from build123d import *

# Parameters (mm, degrees)
ESBO_O1_W                = 15
ESBO_O1_H                = 17
ESBO_O1_R                = 1
RESSALTO_EXTRUS_O1_DEPTH = 1.6
CHANFRO1_SIZE            = 2


with BuildPart() as part:
    # Esboço1 → Ressalto-extrusão1 (new body)
    with BuildSketch(Plane.XY):
        with Locations((2.895389518, -3.7)):
            Rectangle(ESBO_O1_W, ESBO_O1_H)
        with Locations((8.895389518, -3.7)):
            Circle(ESBO_O1_R, mode=Mode.SUBTRACT)
        with Locations((-3.104610482, -3.7)):
            Circle(ESBO_O1_R, mode=Mode.SUBTRACT)
    extrude(amount=RESSALTO_EXTRUS_O1_DEPTH)

    # Chanfro1
    chanfro1_edges = [part.edges().sort_by_distance(p)[0] for p in [
        (-4.604610482, 4.8, 0.8),
        (10.395389518, 4.8, 0.8),
        (10.395389518, -12.2, 0.8),
        (-4.604610482, -12.2, 0.8),
    ]]
    chamfer(chanfro1_edges, length=CHANFRO1_SIZE)


solid = part.part
Geometry check sheet. Reference: the model listing, model coordinates, mm. Round coordinates to 2 decimals unless told otherwise and drop trailing zeros. Order: outer loops, then holes, each group sorted by start corner. A loop starts at its lowest first (then second) coordinate and runs counter-clockwise, first axis right, second up. Notation, with made-up numbers: M 39.25,80.25 L 55.25,80.25 A5 ccw 55.25,88.25 Z; hole C 63.5,31 d6. An arc over 180 degrees is marked long. Answer in a Markdown table with one row per item. Add a question column.
Item 1: Material ranges on L1, parallel to X at y = -3.75, z = 0.4; L2, parallel to Y at x = -3.5, z = 0.1; L3, parallel to Y at x = -2.75, z = 0.35, recorded low to high. Write a range as [from, to].
Item 2: Sectioned sample at B-B, the plane x = 9.5. Enter the section's corners in (y, z).
Item 3: Sectioned sample at C-C, the plane y = -3.7. Enter the section's corners in (x, z).
Item 4: Draft check along Y on faces 1 (the face through (-2.15, -3.4, 0.79)), 2 (the face through (9.409, 3.786, 0.789)), 3 (the face through (3, -4, 0)). Enter one of: released by +Y, released by -Y, zero draft, split by the parting line, or undercut.
Item 5: Sectioned sample at A-A, the plane z = 0.7. Enter the section's corners in (x, y), plus the area to 3 significant figures.
Filled in:
| question | item | result |
|---|---|---|
| 1 | L1 | x = [-4.6, -4.1], [-2.11, 7.9], [9.89, 10.4] |
| 1 | L2 | y = [-11.3, -4.62], [-2.78, 3.9] |
| 1 | L3 | y = [-12.05, -4.64], [-2.76, 4.65] |
| 2 | outline | M -11.1,0 L -4.5,0 L -4.5,1.6 L -11.1,1.6 Z; M -2.9,0 L 3.7,0 L 3.7,1.6 L -2.9,1.6 Z |
| 3 | outline | M -4.6,0 L -4.1,0 L -4.1,1.6 L -4.6,1.6 Z; M -2.1,0 L 7.9,0 L 7.9,1.6 L -2.1,1.6 Z; M 9.9,0 L 10.4,0 L 10.4,1.6 L 9.9,1.6 Z |
| 4 | face 1 | undercut |
| 4 | face 2 | released by +Y |
| 4 | face 3 | zero draft |
| 5 | outline | M -4.6,-10.2 L -2.6,-12.2 L 8.4,-12.2 L 10.4,-10.2 L 10.4,2.8 L 8.4,4.8 L -2.6,4.8 L -4.6,2.8 Z; hole C -3.1,-3.7 d2; hole C 8.9,-3.7 d2 |
| 5 | area | 241 mm² |
